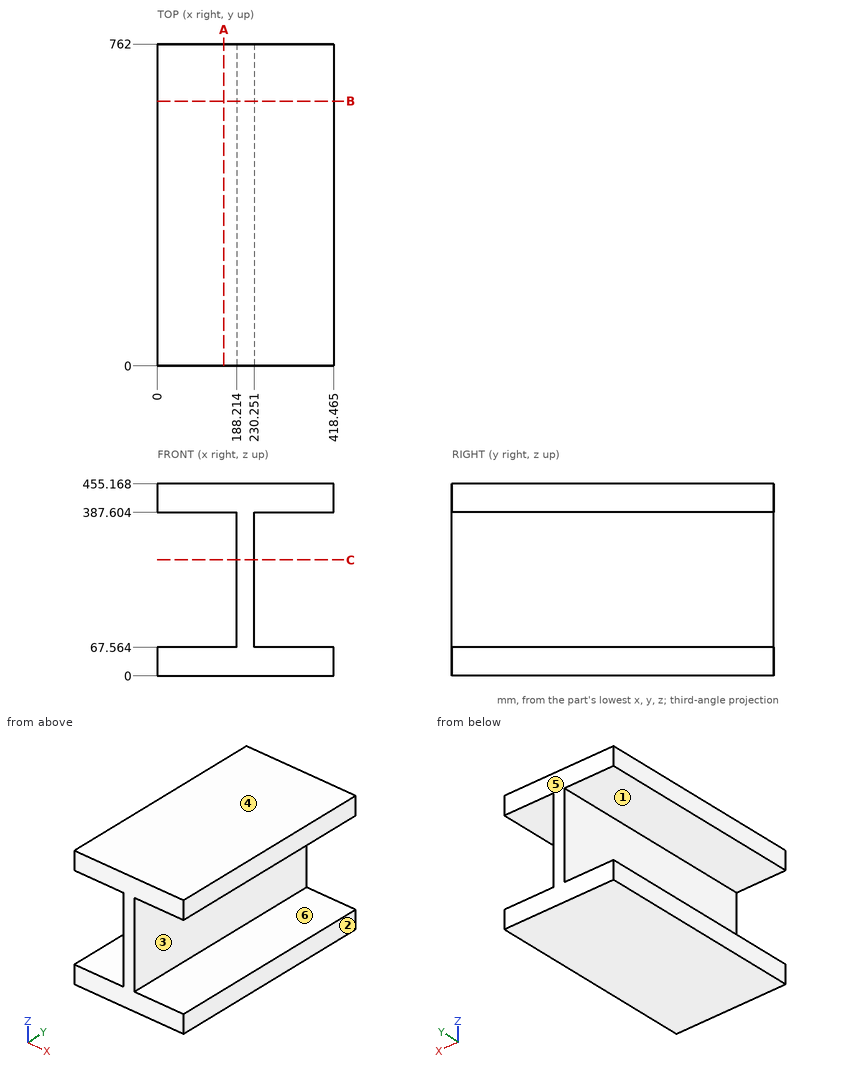
Print and shaded views of the part. All mm, measured from the part's lowest x, y and z. A direction names the side the tool comes from. Give positions to 0.01 mm unless a question says otherwise; leave off trailing zeros. Write each loop counter-clockwise with the first axis right and the second up, starting at its lowest first coordinate (ties: lowest second). Pieces come first, ordered by that corner, then holes. Notation, with made-up numbers: (39.5, 32) -> (78.5, 32) arc R19 cw to (78.5, 57) -> close; hole circle Ø7 at (34.25, 3.5). An arc over 180 degrees is marked (long way). Use CSV: the item, a comma, the result in double quotes. Start each with the question number.
1) Drill centre lines: L1, parallel to Z at x = 160.5, y = 714.5; L2, parallel to X at y = 499.5, z = 372. Where is each one in solid material? Low to high.
2) Two-plate mould, pull along Z, no slides. Class the marked faces 4, 5 and 6: released by +Z, released by -Z, zero draft, split by the parting line, or undercut.
3) Cut at C-C on z = 275. List the corners of the cut face in (x, y).
4) Cut at A-A on x = 158. List the corners of the cut face in (y, z).
5) Tool access for the marked faces 1, 2 and 3: list every direction of +Z, -Z, +X, -X, +Y, -Y with a clear straight run to the whole face (end or side of a thin tool).
6) Cut at B-B on y = 627. List the corners of the cut face in (x, z) (3 decimals), plus the area to 3 significant figures.
7) Pin check, flat tip, straight feed: P1, Ø1.5, axis at y = 575, z = 178, coming from the -X side. Stop position of the tip, or through.
Final values:
1,L1,"z = 0 to 67.56, 387.6 to 455.17"
1,L2,"x = 188.21 to 230.25"
2,face 4,"released by +Z"
2,face 5,"zero draft"
2,face 6,"undercut"
3,outline,"(188.21, 0) -> (230.25, 0) -> (230.25, 762) -> (188.21, 762) -> close"
4,outline,"(0, 0) -> (762, 0) -> (762, 67.56) -> (0, 67.56) -> close; (0, 387.6) -> (762, 387.6) -> (762, 455.17) -> (0, 455.17) -> close"
5,face 1,"-X, +Y, -Y"
5,face 2,"+Z, -Z, +X, +Y, -Y"
5,face 3,"+X, +Y, -Y"
6,outline,"(0, 0) -> (418.465, 0) -> (418.465, 67.564) -> (230.251, 67.564) -> (230.251, 387.604) -> (418.465, 387.604) -> (418.465, 455.168) -> (0, 455.168) -> (0, 387.604) -> (188.214, 387.604) -> (188.214, 67.564) -> (0, 67.564) -> close"
6,area,"70,000 mm2"
7,P1,"stops at x = 188.21"
